from build123d import *

# Parameters (mm, degrees)
F0_W        = 94.615
F0_H        = 65.405
F0_W_2      = 86.9950006521
F0_H_2      = 57.7850006521
F0_R        = 5.08
F0_R_2      = 2.413
F0_W_3      = 15.24
F0_H_3      = 7.62
F0_R_3      = 1.905
F0_R_4      = 2.54
F0_R_5      = 1.143
F0_W_4      = 7.112
F0_H_4      = 1.016
F1_DEPTH    = 4.445
F2_R        = 6.985
F3_SIZE2    = 2.1997045256
F3_SIZE     = 1.27
F3_2_SIZE2  = 2.1997045256
F3_2_SIZE   = 1.27
F4_T        = 2.54
F4_T3_DEPTH = 9.525


# Not quite as in the source:
# - a shell that OpenCascade refuses in one call is made with other operations: the cavity is built on its own and cut out


with BuildPart() as f1:
    # F0 (on Front) → F1 (new body)
    with BuildSketch(Plane.XZ):
        Rectangle(F0_W, F0_H)
        Rectangle(F0_W_2, F0_H_2, mode=Mode.SUBTRACT)
        Rectangle(F0_W_2, F0_H_2)
        with Locations((-34.6075, 0)):
            Circle(F0_R, mode=Mode.SUBTRACT)
        Polygon((24.765, 23.495), (24.765, -23.495), (3.556, -23.495), (-3.556, -23.495), (-24.765, -23.495), (-24.765, 23.495), align=None, mode=Mode.SUBTRACT)
        with Locations((34.6075, 0)):
            Circle(F0_R, mode=Mode.SUBTRACT)
        Polygon((-3.556, -22.479), (3.556, -22.479), (23.749, -22.479), (23.749, 22.479), (-23.749, 22.479), (-23.749, -22.479), align=None)
        with Locations((-19.685, -18.0975)):
            Circle(F0_R_2, mode=Mode.SUBTRACT)
        with Locations((19.685, -18.0975)):
            Circle(F0_R_2, mode=Mode.SUBTRACT)
        with Locations((-12.7, 10.795)):
            Rectangle(F0_W_3, F0_H_3, mode=Mode.SUBTRACT)
        with Locations((-19.685, 18.0975)):
            Circle(F0_R_2, mode=Mode.SUBTRACT)
        with Locations((0, 15.0338392705)):
            Circle(F0_R_3, mode=Mode.SUBTRACT)
        with Locations((12.7, 10.795)):
            Rectangle(F0_W_3, F0_H_3, mode=Mode.SUBTRACT)
        with Locations((19.685, 18.0975)):
            Circle(F0_R_2, mode=Mode.SUBTRACT)
        Polygon((3.556, -23.495), (24.765, -23.495), (24.765, 23.495), (-24.765, 23.495), (-24.765, -23.495), (-3.556, -23.495), (-3.556, -22.479), (-23.749, -22.479), (-23.749, 22.479), (23.749, 22.479), (23.749, -22.479), (3.556, -22.479), align=None)
        with Locations((34.6075, 0)):
            Circle(F0_R)
        with Locations((34.6075, 0)):
            Circle(F0_R_4, mode=Mode.SUBTRACT)
        with Locations((-34.6075, 0)):
            Circle(F0_R)
        with Locations((-34.6075, 0)):
            Circle(F0_R_4, mode=Mode.SUBTRACT)
        with Locations((-19.685, 18.0975)):
            Circle(F0_R_2)
        with Locations((-19.685, 18.0975)):
            Circle(F0_R_5, mode=Mode.SUBTRACT)
        with Locations((-19.685, -18.0975)):
            Circle(F0_R_2)
        with Locations((-19.685, -18.0975)):
            Circle(F0_R_5, mode=Mode.SUBTRACT)
        with Locations((19.685, -18.0975)):
            Circle(F0_R_2)
        with Locations((19.685, -18.0975)):
            Circle(F0_R_5, mode=Mode.SUBTRACT)
        with Locations((19.685, 18.0975)):
            Circle(F0_R_2)
        with Locations((19.685, 18.0975)):
            Circle(F0_R_5, mode=Mode.SUBTRACT)
        with Locations((0, -22.987)):
            Rectangle(F0_W_4, F0_H_4)
        with Locations((-19.685, 18.0975)):
            Circle(F0_R_5)
        with Locations((-19.685, -18.0975)):
            Circle(F0_R_5)
        with Locations((19.685, -18.0975)):
            Circle(F0_R_5)
        with Locations((19.685, 18.0975)):
            Circle(F0_R_5)
    extrude(amount=F1_DEPTH)

    # F2
    f2_edges = [f1.edges().sort_by_distance(p)[0] for p in [
        (-47.3075, -2.2225, 32.7025),
        (-47.3075, -2.2225, -32.7025),
        (47.3075, -2.2225, 32.7025),
        (47.3075, -2.2225, -32.7025),
    ]]
    fillet(f2_edges, radius=F2_R)

    # F3
    f3_edges = [f1.edges().sort_by_distance(p)[0] for p in [
        (-37.1475, -4.445, 0),
    ]]
    f3_side = f1.faces().sort_by_distance((-37.1475, -2.2225, 0))[0]
    chamfer(f3_edges, length=F3_SIZE, length2=F3_SIZE2, reference=f3_side)

    # F3#2
    f3_2_edges = [f1.edges().sort_by_distance(p)[0] for p in [
        (32.0675, -4.445, 0),
    ]]
    f3_2_side = f1.faces().sort_by_distance((32.0675, -2.2225, 0))[0]
    chamfer(f3_2_edges, length=F3_2_SIZE, length2=F3_2_SIZE2, reference=f3_2_side)

    # F4: shell of thickness 2.54, made by hand


with BuildPart() as f4_core1:
    # F4_t2: copy of F1
    add(f1.part)

    # the walls: a layer under each face that stays
    f4_faces = [f4_core1.faces().sort_by_distance(p)[0] for p in [
        (0, -4.445, 0),
        (30.9676477372, -3.81, 0),
        (-38.2473522628, -3.81, 0),
        (0, -2.2225, -32.7025),
        (-45.2616408666, -2.2225, -30.6566408666),
        (45.2616408666, -2.2225, -30.6566408666),
        (-47.3075, -2.2225, 0),
        (47.3075, -2.2225, 0),
        (-45.2616408666, -2.2225, 30.6566408666),
        (45.2616408666, -2.2225, 30.6566408666),
        (0, -2.2225, 32.7025),
        (20.32, -2.2225, 10.795),
        (12.7, -2.2225, 6.985),
        (5.08, -2.2225, 10.795),
        (12.7, -2.2225, 14.605),
        (-12.7, -2.2225, 6.985),
        (-20.32, -2.2225, 10.795),
        (-12.7, -2.2225, 14.605),
        (-5.08, -2.2225, 10.795),
        (-1.905, -2.2225, 15.0338392705),
        (32.0675, -1.5875, 0),
        (-37.1475, -1.5875, 0),
    ]]
    thicken(f4_faces, amount=-F4_T, mode=Mode.SUBTRACT)

    # F4_s4 → F4_t3 (cut)
    with BuildSketch(Plane.XZ.offset(-2.54)):
        Polygon((20.2946, 14.5796), (22.86, 14.605), (22.86, 17.145), (20.32, 17.145), align=None)
        Polygon((20.2946, 7.0104), (22.86, 6.985), (22.86, 4.445), (20.32, 4.445), align=None)
        Polygon((5.1054, 7.0104), (5.08, 4.445), (2.54, 4.445), (2.54, 6.985), align=None)
        Polygon((5.1054, 14.5796), (2.54, 14.605), (2.54, 17.145), (5.08, 17.145), align=None)
        Polygon((-5.1054, 7.0104), (-5.08, 4.445), (-2.54, 4.445), (-2.54, 6.985), align=None)
        Polygon((-20.2946, 7.0104), (-20.32, 4.445), (-22.86, 4.445), (-22.86, 6.985), align=None)
        Polygon((-20.2946, 14.5796), (-22.86, 14.605), (-22.86, 17.145), (-20.32, 17.145), align=None)
        Polygon((-5.1054, 14.5796), (-5.08, 17.145), (-2.54, 17.145), (-2.54, 14.605), align=None)
    extrude(amount=F4_T3_DEPTH, mode=Mode.SUBTRACT)


with BuildPart() as f1_1:
    add(f1.part)

    # what is left inside the walls is the cavity
    f4_cavity = [f4_core1.part.solids().sort_by_distance(p)[0] for p in [
        (0, -0.0254, -10.054167),
    ]]
    add(f4_cavity, mode=Mode.SUBTRACT)


solid = f1_1.part
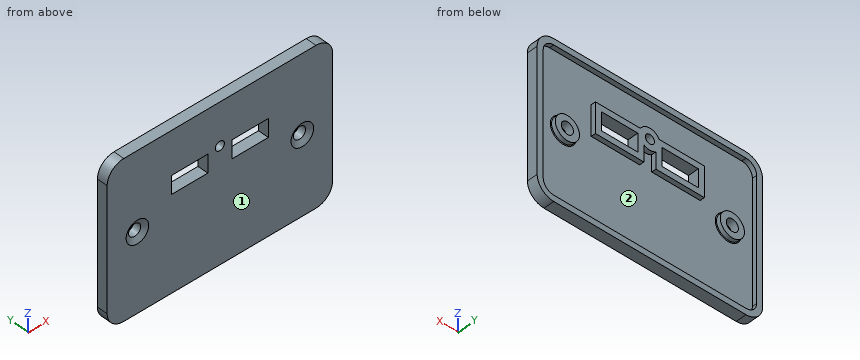
Design review of the part built by this model. Coordinates are the model's own, in mm. Face numbers are marked on the shaded views. Give positions to 0.01 mm unless a question says otherwise; leave off trailing zeros. Order: outer loops, then holes, each group sorted by start corner. A loop starts at its lowest first (then second) coordinate and runs counter-clockwise, first axis right, second up. Notation, with made-up numbers: (58.25, 48) - (82.25, 48) arc R25 ccw to (82.25, 65) - close; hole circle Ø10 at (33, 49). An arc over 180 degrees is marked (long way). Write item = value, one per line. Start each with the question number.
Q1. To check wall thickness, follow L1, parallel to X at y = -2.6, z = 7.5; L2, parallel to Z at x = 0, y = -1.35; L3, parallel to Z at x = 13, y = -3.8 (1 decimal). State the ranges of each line that lie inside material, in increasing order. Write a range as from..to.
Q2. We need section B-B on z = 8. State the section outline as (x, y) points (1 decimal).
Q3. We need section D-D on z = -13. State the section outline as (x, y) points (1 decimal), plus the area to 3 significant figures.
Q4. Clearance check with flat-ended pins moving along their axes: pin 1 Ø6.5 at (x, z) = (-34.61, 0) entering from -Y; pin 2 Ø18 at (x, z) = (-15.5, 13) entering from +Y; pin 3 Ø2 at (x, z) = (-29.5, 4) entering from +Y (3 decimals). State where each tip first meets the part, or that it passes through.
Q5. Mouldability with a two-part tool opening along X and no side actions: class the marked faces 1 and 2 as released by +X, released by -X, zero draft, split by the parting line, or undercut.
Q6. We need section C-C on x = -26. State the section outline as (y, z) points (1 decimal).
Q7. We need section A-A on x = 0. State the section outline as (y, z) points (1 decimal).
Working result:
q1.L1 = -47.31..-20.32, -5.08..5.08, 20.32..47.31
q1.L2 = -32.7..-30.16, 10.59..13.13, 16.94..19.48, 30.16..32.7
q1.L3 = -32.7..7, 14.6..32.7
q2.outline = (-47.3, -4.4) - (-20.3, -4.4) - (-20.3, 0) - (-22.9, 0) - (-22.9, -1.9) - (-44.8, -1.9) - (-44.8, 0) - (-47.3, 0) - close; (-5.1, -4.4) - (5.1, -4.4) - (5.1, 0) - (2.5, 0) - (2.5, -1.9) - (-2.5, -1.9) - (-2.5, 0) - (-5.1, 0) - close; (20.3, -4.4) - (47.3, -4.4) - (47.3, 0) - (44.8, 0) - (44.8, -1.9) - (22.9, -1.9) - (22.9, 0) - (20.3, 0) - close
q3.outline = (-47.3, -4.4) - (47.3, -4.4) - (47.3, 0) - (44.8, 0) - (44.8, -1.9) - (-44.8, -1.9) - (-44.8, 0) - (-47.3, 0) - close
q3.area = 250 mm²
q4.pin_1 = -3.59
q4.pin_2 = 0
q4.pin_3 = -1.905
q5.face_1 = zero draft
q5.face_2 = undercut
q6.outline = (-4.4, -32.7) - (0, -32.7) - (0, -30.2) - (-1.9, -30.2) - (-1.9, 30.2) - (0, 30.2) - (0, 32.7) - (-4.4, 32.7) - close
q7.outline = (-4.4, -32.7) - (0, -32.7) - (0, -30.2) - (-1.9, -30.2) - (-1.9, 10.6) - (0, 10.6) - (0, 13.1) - (-4.4, 13.1) - close; (-4.4, 16.9) - (0, 16.9) - (0, 19.5) - (-1.9, 19.5) - (-1.9, 30.2) - (0, 30.2) - (0, 32.7) - (-4.4, 32.7) - close
